Design review of the part shown in the three views and the two pictorial views. Dimensions are in mm from the part's minimum x, y and z. Round coordinates to 2 decimals unless told otherwise and drop trailing zeros. Loops run counter-clockwise (first coordinate to the right, second up) from the corner with the lowest first, then second, coordinate; pieces in that order, holes last. Notation, with made-up numbers: M 52.5,-25.5 L 90.5,-25.5 A35 ccw 90.5,8.5 Z; hole C -1.5,-14.5 d5. An arc over 180 degrees is marked long. Return JSON: item names as keys, results as strings. Group by question number.
Q1. Consider section C-C (x = 55). State the section outline as (y, z) points, and give its area (3 significant figures).
Q2. To check wall thickness, follow line 1 along Y through (x, z) = (10, 1.6); line 2 along Y through (x, z) = (55, 0.8). State the ranges of each line that lie inside material, in increasing order.
Q3. Clearance check with a flat-ended pin moving along its axis: pin 1 Ø6.5 at (x, y) = (10, 32.5) entering from +Z. State where the tip first meets the part, or that it passes through.
Q4. Consider section B-B (z = 1). State the section outline as (x, y) points, and give its area (3 significant figures).
Q5. Consider section D-D (x = 9). State the section outline as (y, z) points.
Q6. Consider section A-A (y = 8.5). State the section outline as (x, z) points, and give its area (3 significant figures).
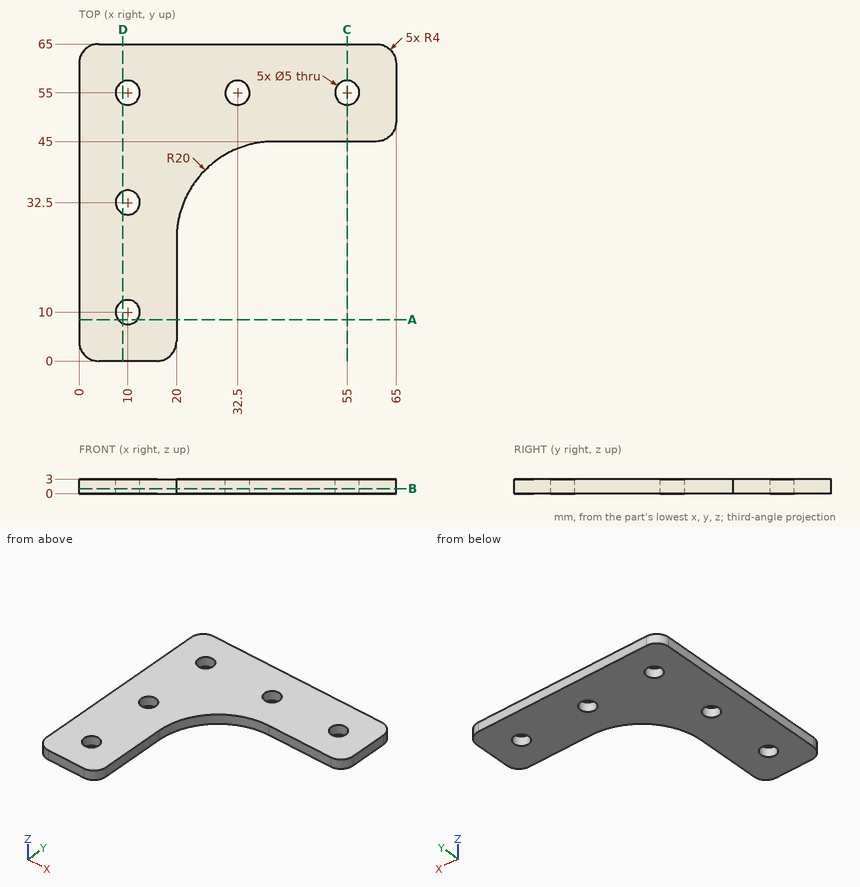
Values:
{
 "1": {"outline": "M 45,0 L 52.5,0 L 52.5,3 L 45,3 Z; M 57.5,0 L 65,0 L 65,3 L 57.5,3 Z", "area": "45.0 mm2"},
 "2": {"line 1": "y = 0 to 7.5, 12.5 to 30, 35 to 52.5, 57.5 to 65", "line 2": "y = 45 to 52.5, 57.5 to 65"},
 "3": {"pin 1": "stops at z = 3"},
 "4": {"outline": "M 0,4 A4 ccw 4,0 L 16,0 A4 ccw 20,4 L 20,25 A20 cw 40,45 L 61,45 A4 ccw 65,49 L 65,61 A4 ccw 61,65 L 4,65 A4 ccw 0,61 Z; hole C 10,10 d5; hole C 10,32.5 d5; hole C 10,55 d5; hole C 32.5,55 d5; hole C 55,55 d5", "area": "2,170 mm2"},
 "5": {"outline": "M 0,0 L 7.71,0 L 7.71,3 L 0,3 Z; M 12.29,0 L 30.21,0 L 30.21,3 L 12.29,3 Z; M 34.79,0 L 52.71,0 L 52.71,3 L 34.79,3 Z; M 57.29,0 L 65,0 L 65,3 L 57.29,3 Z"},
 "6": {"outline": "M 0,0 L 8,0 L 8,3 L 0,3 Z; M 12,0 L 20,0 L 20,3 L 12,3 Z", "area": "48.0 mm2"}
}
